Check sheet for the modelled part. Datum: model origin and axes. Units: mm. A direction names the side the tool comes from. Give positions to 0.01 mm unless a question says otherwise; leave off trailing zeros. Order: outer loops, then holes, each group sorted by start corner. A loop starts at its lowest first (then second) coordinate and runs counter-clockwise, first axis right, second up. Notation, with made-up numbers: (1.5, -35) - (13.5, -35) arc R16 ccw to (13.5, -14) - close; hole circle Ø10 at (22.25, 18). An arc over 180 degrees is marked (long way). Answer in a Markdown table with one row per item.
from build123d import *

# Parameters (mm, degrees)
BOSS_EXTRUDE1_DEPTH       = 3.175
F_4_CLEARANCE_HOLE1_D     = 2.9464
F_4_CLEARANCE_HOLE1_DEPTH = 3.302
F_4_CLEARANCE_HOLE1_TIP   = 0.885187864
FILLET1_R                 = 6.35


with BuildPart() as part:
    # Sketch1 → Boss-Extrude1 (new body)
    with BuildSketch(Plane.XY):
        Polygon((-15.08125, -3.0353), (-15.08125, -17.4625), (-24.60625, -17.4625), (-24.60625, 4.7625), (-9.525, 4.7625), (-9.525, 50.8), (9.525, 50.8), (9.525, 4.7625), (24.60625, 4.7625), (24.60625, -17.4625), (15.08125, -17.4625), (15.08125, -3.0353), align=None)
    extrude(amount=BOSS_EXTRUDE1_DEPTH)

    # #4 Clearance Hole1
    with Locations(Plane.XY.offset(3.175)):
        with Locations((-19.84375, 0), (19.84375, 0), (19.84375, -12.7), (-19.84375, -12.7)):
            Hole(F_4_CLEARANCE_HOLE1_D / 2, depth=F_4_CLEARANCE_HOLE1_DEPTH)
            with Locations((0, 0, -(F_4_CLEARANCE_HOLE1_DEPTH + F_4_CLEARANCE_HOLE1_TIP / 2))):  # 118° drill point
                Cone(0, F_4_CLEARANCE_HOLE1_D / 2, F_4_CLEARANCE_HOLE1_TIP, mode=Mode.SUBTRACT)

    # Fillet1
    fillet1_edges = [part.edges().sort_by_distance(p)[0] for p in [
        (-9.525, 4.7625, 1.5875),
        (9.525, 4.7625, 1.5875),
    ]]
    fillet(fillet1_edges, radius=FILLET1_R)


solid = part.part
(1) Gauge pin test, flat ends, axial feed: P1, Ø2.5, axis at x = 19.84, y = -12.7, coming from the +Z side; P2, Ø1.6, axis at y = 28.5, z = 1, coming from the +X side (3 decimals); P3, Ø1, axis at x = -21.5, z = 1.5, coming from the +Y side; P4, Ø1.5, axis at x = -7, y = 9.5, coming from the -Z side. Record the tip position at first contact, or that the pin passes through.
Geometry says:
| item | result |
|---|---|
| P1 | through |
| P2 | x = 9.525 |
| P3 | y = 4.76 |
| P4 | z = 0 |
(2) Thickness scan on L1, parallel to X at y = -6, z = 1.2; L2, parallel to Y at x = -22, z = 2.8; L3, parallel to Y at x = -7.5, z = 3.05. Record the ranges inside material, lowest first.
Geometry says:
| item | result |
|---|---|
| L1 | -24.61 to -15.08, 15.08 to 24.61 |
| L2 | -17.46 to 4.76 |
| L3 | -3.04 to 50.8 |
(3) Access from +Z, -Z, +X, -X, +Y, -Y to the whole of each face (thin tool, end or side, straight path). Record for faces 4 (the flat face through (9.525, 31, 2)), 5 (the flat face through (-15.081, -10, 2)), 6 (the flat face through (-9.525, 31, 2)).
Geometry says:
| item | result |
|---|---|
| face 4 | +Z, -Z, +X, +Y |
| face 5 | +Z, -Z, -Y |
| face 6 | +Z, -Z, -X, +Y |
(4) Mould release check, pull along Y, two halves, no side actions. Record for faces 1 (the cylindrical face through (-21.205, -0.564, 1.565)), 2 (the flat face through (-24.606, -7, 2)), 3 (the flat face through (-20, 4.762, 2)): pulls with the +Y half, pulls with the -Y half, needs draft (parallel to the pull), parting line crosses it, or undercut.
Geometry says:
| item | result |
|---|---|
| face 1 | undercut |
| face 2 | needs draft |
| face 3 | pulls with the +Y half |
(5) Cross-section at D-D, the plane x = -17. Record the cut outline in (y, z) (1 decimal), then the cut area to 3 significant figures.
Geometry says:
| item | result |
|---|---|
| outline | (-17.5, 0) - (4.8, 0) - (4.8, 3.2) - (-17.5, 3.2) - close |
| area | 70.6 mm² |
(6) Cross-section at B-B, the plane z = 1.7. Give the number of separate pieces and of enclosed holes in the cut face, then the cut area to 3 significant figures.
Geometry says:
| item | result |
|---|---|
| separate pieces | 1 |
| enclosed holes | 4 |
| area | 1,530 mm² |
(7) Cross-section at C-C, the plane y = 0. Record the cut outline in (x, z) (3 decimals), then the cut area to 3 significant figures.
Geometry says:
| item | result |
|---|---|
| outline | (-24.606, 0) - (-21.317, 0) - (-21.317, 3.175) - (-24.606, 3.175) - close; (-18.371, 0) - (18.371, 0) - (18.371, 3.175) - (-18.371, 3.175) - close; (21.317, 0) - (24.606, 0) - (24.606, 3.175) - (21.317, 3.175) - close |
| area | 138 mm² |
(8) Cross-section at A-A, the plane y = -12.7. Record the cut outline in (x, z) (3 decimals).
Geometry says:
| item | result |
|---|---|
| outline | (-24.606, 0) - (-21.317, 0) - (-21.317, 3.175) - (-24.606, 3.175) - close; (-18.371, 0) - (-15.081, 0) - (-15.081, 3.175) - (-18.371, 3.175) - close; (15.081, 0) - (18.371, 0) - (18.371, 3.175) - (15.081, 3.175) - close; (21.317, 0) - (24.606, 0) - (24.606, 3.175) - (21.317, 3.175) - close |
